Here's how the part is built. I have some questions about the finished solid (model axes, mm). Coordinates: 2 decimals unless noted, no trailing zeros. Loops run counter-clockwise (first coordinate to the right, second up) from the corner with the lowest first, then second, coordinate; pieces in that order, holes last.
```python
from build123d import *

# Parameters (mm, degrees)
F0_W     = 165.1
F0_H     = 292.1
F1_DEPTH = 4.7625
F3_D     = 6.7564
F4_W     = 120
F4_H     = 46
F4_H_2   = 26.5
F5_DEPTH = 4.7635


with BuildPart() as f1:
    # F0 (on Front) → F1 (new body)
    with BuildSketch(Plane.XZ):
        with Locations((82.55, 146.05)):
            Rectangle(F0_W, F0_H)
    extrude(amount=F1_DEPTH)

    # F3 (through all)
    with Locations(Plane.XZ.offset(4.7625)):
        with Locations((12.7, 279.4), (152.4, 279.4), (12.7, 12.7), (152.4, 12.7)):
            Hole(F3_D / 2)

    # F4 (on face) → F5 (cut, through all)
    with BuildSketch(Plane.XZ.offset(4.7625)):
        with Locations((82.5, 231.1)):
            Rectangle(F4_W, F4_H)
        with Locations((82.5, 156.85)):
            Rectangle(F4_W, F4_H_2)
    extrude(amount=-F5_DEPTH, mode=Mode.SUBTRACT)


solid = f1.part
```
1. I need wall thicknesses on line 1 along Z through (x, y) = (107, -2.6); line 2 along Z through (x, y) = (152.4, -2.1); line 3 along X through (y, z) = (-2.6, 279.4). Which ranges of each line are inside material? Lowest first, please.
2. I want a section at D-D (y = -2.55). Please give me the cut outline in (x, z).
3. I want a section at C-C (z = 279.4). Please give me the cut outline in (x, y), then the cut area to 3 significant figures.
4. I want a section at A-A (z = 221). Please give me the cut outline in (x, y), then the cut area to 3 significant figures.
5. For pin 1 (4 mm diameter, centred on x = 12.7, z = 279.4, fed in from -Y), with a flat end and sliding along its axis, tell me the tip position at first contact or that it passes through.
6. I want a section at B-B (x = 60). Please give me the cut outline in (y, z).
7. We'd pull the mould along Z, two halves only. Please class faces 1 (the flat face through (81, -4.762, 116)), 2 (the cylindrical face through (13.14, -2.35, 282.75)), 3 (the cylindrical face through (15.381, -2.348, 10.644)): +Z half, -Z half, draft (parallel to the pull), parting line (faces both ways), or undercut.
Response values:
1. line 1: z = 0 to 143.6, 170.1 to 208.1, 254.1 to 292.1
1. line 2: z = 0 to 9.32, 16.08 to 276.02, 282.78 to 292.1
1. line 3: x = 0 to 9.32, 16.08 to 149.02, 155.78 to 165.1
2. outline: (0, 0) - (165.1, 0) - (165.1, 292.1) - (0, 292.1) - close; hole circle Ø6.76 at (12.7, 12.7); hole circle Ø6.76 at (12.7, 279.4); hole (22.5, 143.6) - (142.5, 143.6) - (142.5, 170.1) - (22.5, 170.1) - close; hole (22.5, 208.1) - (142.5, 208.1) - (142.5, 254.1) - (22.5, 254.1) - close; hole circle Ø6.76 at (152.4, 12.7); hole circle Ø6.76 at (152.4, 279.4)
3. outline: (0, -4.76) - (9.32, -4.76) - (9.32, 0) - (0, 0) - close; (16.08, -4.76) - (149.02, -4.76) - (149.02, 0) - (16.08, 0) - close; (155.78, -4.76) - (165.1, -4.76) - (165.1, 0) - (155.78, 0) - close
3. area: 722 mm2
4. outline: (0, -4.76) - (22.5, -4.76) - (22.5, 0) - (0, 0) - close; (142.5, -4.76) - (165.1, -4.76) - (165.1, 0) - (142.5, 0) - close
4. area: 215 mm2
5. pin 1: passes through
6. outline: (-4.76, 0) - (0, 0) - (0, 143.6) - (-4.76, 143.6) - close; (-4.76, 170.1) - (0, 170.1) - (0, 208.1) - (-4.76, 208.1) - close; (-4.76, 254.1) - (0, 254.1) - (0, 292.1) - (-4.76, 292.1) - close
7. face 1: draft
7. face 2: undercut
7. face 3: undercut
